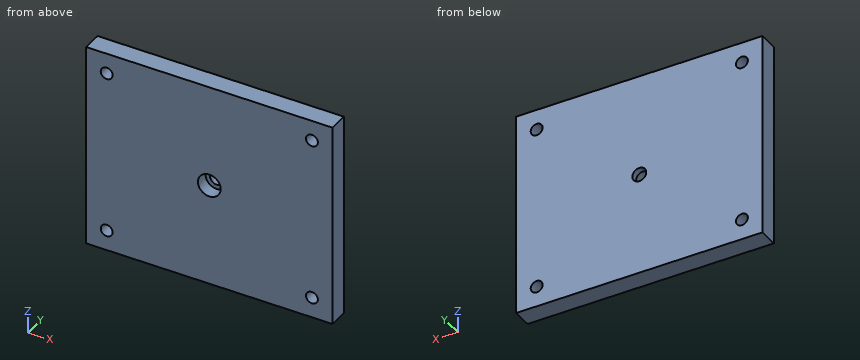
```python
from build123d import *

# Parameters (mm, degrees)
SKETCH1_W                                        = 120
SKETCH1_H                                        = 100
BOSS_EXTRUDE1_DEPTH                              = 9.525
M5_CLEARANCE_HOLE1_D                             = 5.8
CBORE_FOR_1_4_SOCKET_HEAD_CAP_SCREW1_D           = 6.7564
CBORE_FOR_1_4_SOCKET_HEAD_CAP_SCREW1_CBORE_D     = 11.1125
CBORE_FOR_1_4_SOCKET_HEAD_CAP_SCREW1_CBORE_DEPTH = 6.35


with BuildPart() as part:
    # Sketch1 → Boss-Extrude1 (new body)
    with BuildSketch(Plane(origin=(0, 0, 0), x_dir=(1, 0, 0), z_dir=(0, 1, 0))):
        Rectangle(SKETCH1_W, SKETCH1_H)
    extrude(amount=BOSS_EXTRUDE1_DEPTH)

    # M5 Clearance Hole1 (through all)
    with Locations(Plane(origin=(0, 9.525, 0), x_dir=(1, 0, 0), z_dir=(0, 1, 0))):
        with Locations((-50, -40), (-50, 40), (50, 40), (50, -40)):
            Hole(M5_CLEARANCE_HOLE1_D / 2)

    # CBORE for 1/4 Socket Head Cap Screw1 (through all)
    with Locations(Plane(origin=(0, 0, 0), x_dir=(-1, 0, 0), z_dir=(0, -1, 0))):
        with Locations((0, 0)):
            CounterBoreHole(CBORE_FOR_1_4_SOCKET_HEAD_CAP_SCREW1_D / 2, CBORE_FOR_1_4_SOCKET_HEAD_CAP_SCREW1_CBORE_D / 2, CBORE_FOR_1_4_SOCKET_HEAD_CAP_SCREW1_CBORE_DEPTH)


solid = part.part
```
The listing builds one solid part. Answer for the finished solid, in the listing's coordinates (mm). Round coordinates to 2 decimals unless told otherwise and drop trailing zeros. Order: outer loops, then holes, each group sorted by start corner. A loop starts at its lowest first (then second) coordinate and runs counter-clockwise, first axis right, second up. Notation, with made-up numbers: (6, 79) - (10, 79) arc R22 cw to (10, 97) - close; hole circle Ø9 at (-14.75, 1.5). An arc over 180 degrees is marked (long way). Put each result on its own line as item: value. Start each with the question number.
(1) Straight lines are drawn through the part: probe 1 along Z at (x, y) = (50, 6.5); probe 2 along X at (y, z) = (2.5, -40); probe 3 along Z at (x, y) = (0, 2.25). For each, find the intervals that lie inside material, in ascending order. Write a range as from..to.
(2) Find section A-A (x = 50). Give the vertices of the cut face in (y, z) (3 decimals).
(3) Find section C-C (y = 5). Give the vertices of the cut face in (x, z), plus the area to 3 significant figures.
(4) Given P1, Ø10, axis at x = 0, z = 0, coming from the -Y side, flat-ended and moving along its own axis, determine where the tip first touches the part or whether it passes through.
(5) Find section B-B (z = 40). Give the vertices of the cut face in (x, y) (3 decimals), plus the area to 3 significant figures.
(6) Find section D-D (z = 0). Give the vertices of the cut face in (x, y) (3 decimals), plus the area to 3 significant figures.
Reply:
1. probe 1: -50..-42.9, -37.1..37.1, 42.9..50
1. probe 2: -60..-52.9, -47.1..47.1, 52.9..60
1. probe 3: -50..-5.56, 5.56..50
2. outline: (0, -50) - (9.525, -50) - (9.525, -42.9) - (0, -42.9) - close; (0, -37.1) - (9.525, -37.1) - (9.525, 37.1) - (0, 37.1) - close; (0, 42.9) - (9.525, 42.9) - (9.525, 50) - (0, 50) - close
3. outline: (-60, -50) - (60, -50) - (60, 50) - (-60, 50) - close; hole circle Ø5.8 at (-50, -40); hole circle Ø5.8 at (-50, 40); hole circle Ø11.11 at (0, 0); hole circle Ø5.8 at (50, -40); hole circle Ø5.8 at (50, 40)
3. area: 11,800 mm^2
4. P1: y = 6.35
5. outline: (-60, 0) - (-52.9, 0) - (-52.9, 9.525) - (-60, 9.525) - close; (-47.1, 0) - (47.1, 0) - (47.1, 9.525) - (-47.1, 9.525) - close; (52.9, 0) - (60, 0) - (60, 9.525) - (52.9, 9.525) - close
5. area: 1,030 mm^2
6. outline: (-60, 0) - (-5.556, 0) - (-5.556, 6.35) - (-3.378, 6.35) - (-3.378, 9.525) - (-60, 9.525) - close; (3.378, 6.35) - (5.556, 6.35) - (5.556, 0) - (60, 0) - (60, 9.525) - (3.378, 9.525) - close
6. area: 1,050 mm^2
